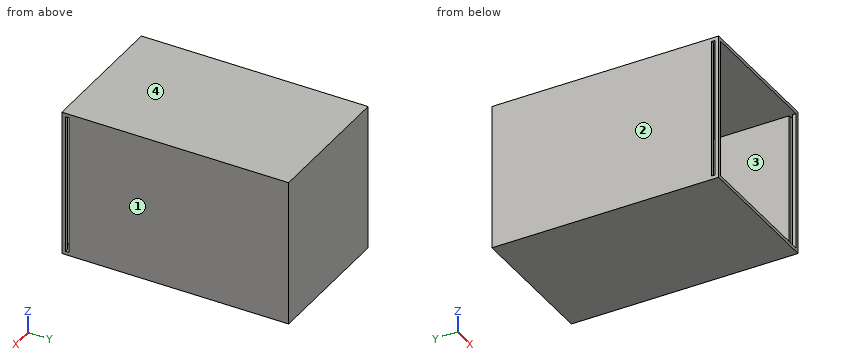
```python
from build123d import *

# Parameters (mm, degrees)
F0_W     = 127
F0_H     = 127
F1_DEPTH = 3.175
F2_W     = 3.175
F2_H     = 127
F3_DEPTH = 203.2
F4_W     = 127
F4_H     = 206.375
F5_DEPTH = 3.175
F6_W     = 127
F6_H     = 206.375
F7_DEPTH = 3.175
F8_W     = 3.175
F8_H     = 127
F9_DEPTH = 127.001


with BuildPart() as f1:
    # F0 (on Front) → F1 (new body)
    with BuildSketch(Plane.XZ):
        Rectangle(F0_W, F0_H)
    extrude(amount=F1_DEPTH)

    # F2 (on face) → F3 (join)
    with BuildSketch(Plane.XZ.offset(3.175)):
        with Locations((-61.9125, 0)):
            Rectangle(F2_W, F2_H)
        with Locations((61.9125, 0)):
            Rectangle(F2_W, F2_H)
    extrude(amount=F3_DEPTH)

    # F4 (on face) → F5 (join)
    with BuildSketch(Plane.XY.offset(63.5)):
        with Locations((0, -103.1875)):
            Rectangle(F4_W, F4_H)
    extrude(amount=F5_DEPTH)

    # F6 (on face) → F7 (join)
    with BuildSketch(Plane(origin=(0, 0, -63.5), x_dir=(1, 0, 0), z_dir=(0, 0, -1))):
        with Locations((0, 103.1875)):
            Rectangle(F6_W, F6_H)
    extrude(amount=F7_DEPTH)

    # F8 (on face) → F9 (cut, through all)
    with BuildSketch(Plane.YZ.offset(63.5)):
        with Locations((-201.6125, 0)):
            Rectangle(F8_W, F8_H)
    extrude(amount=-F9_DEPTH, mode=Mode.SUBTRACT)


solid = f1.part
```
Design review of the part built by this model. Coordinates are the model's own, in mm. Face numbers are marked on the shaded views. Coordinates: 2 decimals unless noted, no trailing zeros. Order: outer loops, then holes, each group sorted by start corner. A loop starts at its lowest first (then second) coordinate and runs counter-clockwise, first axis right, second up.
1) Wall thickness on line 1 along X through (y, z) = (-77, -42.5) (3 decimals); line 2 along Z through (x, y) = (-26, -41) (3 decimals); line 3 along Y through (x, z) = (-41.5, 16) (3 decimals): over which ranges is each line inside the solid? List them lowest first.
2) Take a section at B-B, the plane y = -126. Give the boundary of the cut face in (x, z) (3 decimals), and give its area (3 significant figures).
3) Clearance check with a flat-ended pin moving along its axis: pin 1 (6 mm diameter, centred on x = -2, z = -5, fed in from -Y) (3 decimals). State where the tip first meets the part, or that it passes through.
4) Mouldability with a two-part tool opening along X and no side actions: class the marked faces 1, 2, 3 and 4 as +X half, -X half, draft (parallel to the pull), parting line (faces both ways), or undercut.
5) Take a section at A-A, the plane z = 3. Give the boundary of the cut face in (x, y) (3 decimals).
6) Take a section at C-C, the plane x = 48. Give the boundary of the cut face in (y, z) (3 decimals).
Returned:
1. line 1: x = -63.5 to -60.325, 60.325 to 63.5
1. line 2: z = -66.675 to -63.5, 63.5 to 66.675
1. line 3: y = -3.175 to 0
2. outline: (-63.5, -66.675) - (63.5, -66.675) - (63.5, 66.675) - (-63.5, 66.675) - close; hole (-60.325, -63.5) - (60.325, -63.5) - (60.325, 63.5) - (-60.325, 63.5) - close
2. area: 1,610 mm2
3. pin 1: stops at y = -3.175
4. face 1: +X half
4. face 2: -X half
4. face 3: undercut
4. face 4: draft
5. outline: (-63.5, -206.375) - (-60.325, -206.375) - (-60.325, -203.2) - (-63.5, -203.2) - close; (-63.5, -200.025) - (-60.325, -200.025) - (-60.325, -3.175) - (60.325, -3.175) - (60.325, -200.025) - (63.5, -200.025) - (63.5, 0) - (-63.5, 0) - close; (60.325, -206.375) - (63.5, -206.375) - (63.5, -203.2) - (60.325, -203.2) - close
6. outline: (-206.375, -66.675) - (0, -66.675) - (0, 66.675) - (-206.375, 66.675) - (-206.375, 63.5) - (-3.175, 63.5) - (-3.175, -63.5) - (-206.375, -63.5) - close
